Part model, mm, in its own coordinate system. A direction names the side the tool comes from. Give positions to 0.01 mm unless a question says otherwise; leave off trailing zeros. Order: outer loops, then holes, each group sorted by start corner. A loop starts at its lowest first (then second) coordinate and runs counter-clockwise, first axis right, second up. Notation, with made-up numbers: M 53,-5.75 L 86,-5.75 A20 ccw 86,10.25 Z; hole C 25.5,75 d3. An arc over 180 degrees is marked long. Return JSON: item names as keys, results as strings.
from build123d import *

# Parameters (mm, degrees)
SKETCH_1_W               = 49.93556627
SKETCH_1_H               = 8
EXTRUDE_1_DEPTH          = 58
SKETCH_2_R               = 2.5
SKETCH_2_R_2             = 1.5
CUT_EXTRUDE_1_DEPTH      = 10
CUT_EXTRUDE_2_DEPTH      = 53
CUT_EXTRUDE_2_DEPTH_BACK = 7
SKETCH_3_R               = 1.5
CHAMFER_1_SIZE           = 1.5


with BuildPart() as part:
    # 草图1 → 凸台-拉伸1 (new body)
    with BuildSketch(Plane.XY):
        with Locations((0, 106)):
            Rectangle(SKETCH_1_W, SKETCH_1_H)
    extrude(amount=EXTRUDE_1_DEPTH)

    # 草图2 → 切除-拉伸1 (cut)
    with BuildSketch(Plane(origin=(0, 110, 0), x_dir=(1, 0, 0), z_dir=(0, 1, 0))):
        with Locations(Location((0, -29, 0), (0, 0, 270))):
            Circle(SKETCH_2_R)
        with Locations(Location((0, -39, 0), (0, 0, 270))):
            Circle(SKETCH_2_R_2)
        with Locations(Location((0, -19, 0), (0, 0, 270))):
            Circle(SKETCH_2_R_2)
        with BuildLine():
            Line((24.967783135, -53), (10.967783135, -53))
            ThreePointArc((10.967783135, -53), (8.846462792, -52.121320344), (7.967783135, -50))
            Line((7.967783135, -50), (7.967783135, -8))
            ThreePointArc((7.967783135, -8), (8.846462792, -5.878679656), (10.967783135, -5))
            Line((10.967783135, -5), (24.967783135, -5))
            Line((24.967783135, -5), (24.967783135, -53))
        make_face()
        with BuildLine():
            Line((-7.967783135, -50), (-7.967783135, -8))
            ThreePointArc((-7.967783135, -8), (-8.846462792, -5.878679656), (-10.967783135, -5))
            Line((-10.967783135, -5), (-24.967783135, -5))
            Line((-24.967783135, -5), (-24.967783135, -53))
            Line((-24.967783135, -53), (-10.967783135, -53))
            ThreePointArc((-10.967783135, -53), (-8.846462792, -52.121320344), (-7.967783135, -50))
        make_face()
    extrude(amount=-CUT_EXTRUDE_1_DEPTH, mode=Mode.SUBTRACT)

    # 草图3 → 切除-拉伸2 (cut, two sides: drawn at the far end of the back side and taken through both)
    with BuildSketch(Plane.XY.offset(5).offset(-CUT_EXTRUDE_2_DEPTH_BACK)):
        with Locations(Location((18.967783135, 106, 0), (0, 0, 180))):
            Circle(SKETCH_3_R)
        with Locations(Location((-18.967783135, 106, 0), (0, 0, 180))):
            Circle(SKETCH_3_R)
    extrude(amount=CUT_EXTRUDE_2_DEPTH + CUT_EXTRUDE_2_DEPTH_BACK, mode=Mode.SUBTRACT)

    # 倒角1
    chamfer_1_edges = [part.edges().sort_by_distance(p)[0] for p in [
        (0, 102, 17.5),
        (0, 102, 37.5),
    ]]
    chamfer(chamfer_1_edges, length=CHAMFER_1_SIZE)


solid = part.part
Q1. Band-saw the part on A-A (x = 0). Give the cut face in (y, z).
Established:
{"outline": "M 102,0 L 110,0 L 110,17.5 L 103.5,17.5 L 102,16 Z; M 102,22 L 103.5,20.5 L 110,20.5 L 110,26.5 L 102,26.5 Z; M 102,31.5 L 110,31.5 L 110,37.5 L 103.5,37.5 L 102,36 Z; M 102,42 L 103.5,40.5 L 110,40.5 L 110,58 L 102,58 Z"}
Q2. Probe line 1 along X through (y, z) = (106, 55.5); line 2 along Z through (x, y) = (12, 107); line 3 along Z through (x, y) = (-1, 105). List the from-to ranges inside material, lowest first.
Established:
{"line 1": "x = -24.97 to -20.47, -17.47 to 17.47, 20.47 to 24.97", "line 2": "z = 0 to 5, 53 to 58", "line 3": "z = 0 to 17.88, 20.12 to 26.71, 31.29 to 37.88, 40.12 to 58"}
Q3. 3-axis set-ups, long thin cutter, end or side, ignore diameter. For faces 4 (the cylindrical face through (-8.87, 106.056, 52.145)), 5 (the cylindrical face through (-0.9, 106.8, 37.8)), 6 (the cylindrical face through (8.87, 106.056, 52.145)): which of +Z, -Z, +X, -X, +Y, -Y reach the whole face in a straight line?
Established:
{"face 4": "-X, +Y, -Y", "face 5": "+Y, -Y", "face 6": "+X, +Y, -Y"}
Q4. Pin check, flat tips, straight feed: pin 1 (4 mm diameter, centred on x = 0, z = 19, fed in from -Y); pin 2 (2.5 mm diameter, centred on x = -18.97, y = 106, fed in from -Z) (1 decimal). Stop position of each tip, or through.
Established:
{"pin 1": "stops at y = 103", "pin 2": "passes through"}
Q5. Two-plate mould, pull along Z, no slides. Class faces 1 (the flat face through (0, 106, 58)), 2 (the flat face through (-24.968, 106, 55)), 3 (the cylindrical face through (-8.823, 106.056, 5.902)): +Z half, -Z half, draft (parallel to the pull), parting line (faces both ways), or undercut.
Established:
{"face 1": "+Z half", "face 2": "draft", "face 3": "undercut"}
Q6. Band-saw the part on C-C (y = 109). Give the cut face in (x, z).
Established:
{"outline": "M -24.97,0 L 24.97,0 L 24.97,5 L 10.97,5 A3 cw 7.97,8 L 7.97,50 A3 cw 10.97,53 L 24.97,53 L 24.97,58 L -24.97,58 L -24.97,53 L -10.97,53 A3 cw -7.97,50 L -7.97,8 A3 cw -10.97,5 L -24.97,5 Z; hole C 0,29 d5; hole C 0,19 d3; hole C 0,39 d3"}
Q7. Band-saw the part on D-D (z = 51). Give the cut face in (x, y), then the cut area to 3 significant figures.
Established:
{"outline": "M -8.14,102 L 8.14,102 L 8.14,110 L -8.14,110 Z", "area": "130 mm²"}
Q8. Band-saw the part on B-B (z = 29). Give the cut face in (x, y), then the cut area to 3 significant figures.
Established:
{"outline": "M -7.97,102 L -2.5,102 L -2.5,110 L -7.97,110 Z; M 2.5,102 L 7.97,102 L 7.97,110 L 2.5,110 Z", "area": "87.5 mm²"}
